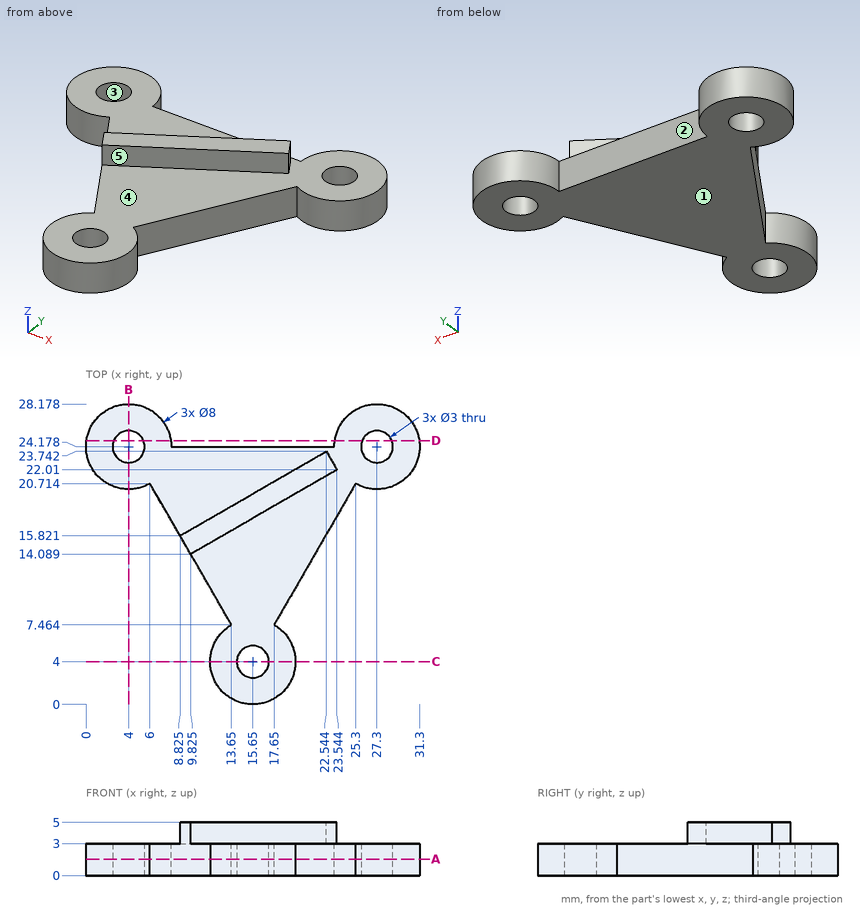
Geometry: see drawing. Coordinates: mm, zero at the bounding-box minimum. A direction names the side the tool comes from. Coordinates: 2 decimals unless noted, no trailing zeros. Loops run counter-clockwise (first coordinate to the right, second up) from the corner with the lowest first, then second, coordinate; pieces in that order, holes last. Notation, with made-up numbers: (50, 11) -> (83, 11) arc R3 ccw to (83, 16) -> close; hole circle Ø10 at (-30.75, 28). An arc over 180 degrees is marked (long way). Use a Markdown table: item, result.
1) Pull-direction query (X, two-part tool) for the marked faces 3, 4 and 5; classes: released by +X, released by -X, zero draft, split by the parting line, or undercut.
Results found:
| item | result |
|---|---|
| face 3 | undercut |
| face 4 | zero draft |
| face 5 | released by +X |
2) Cut plane C-C (y = 4). Return the cut outline in (x, z).
Results found:
| item | result |
|---|---|
| outline | (11.65, 0) -> (14.15, 0) -> (14.15, 3) -> (11.65, 3) -> close; (17.15, 0) -> (19.65, 0) -> (19.65, 3) -> (17.15, 3) -> close |
3) Cut plane A-A (z = 1.55). Give the number of separate pieces and of enclosed holes in the cut face.
Results found:
| item | result |
|---|---|
| separate pieces | 1 |
| enclosed holes | 3 |
4) Cut plane D-D (y = 24.75). Return the cut outline in (x, z).
Results found:
| item | result |
|---|---|
| outline | (0.04, 0) -> (2.61, 0) -> (2.61, 3) -> (0.04, 3) -> close; (5.39, 0) -> (7.96, 0) -> (7.96, 3) -> (5.39, 3) -> close; (23.34, 0) -> (25.91, 0) -> (25.91, 3) -> (23.34, 3) -> close; (28.69, 0) -> (31.26, 0) -> (31.26, 3) -> (28.69, 3) -> close |
5) Contact query for flat-ended pins moving along their axis: pin 1 (1.5 mm diameter, centred on y = 22, z = 1.5, fed in from +X); pin 2 (3 mm diameter, centred on y = 8.5, z = 3.5, fed in from +X) (1 decimal). Output: stop coordinate, or through.
Results found:
| item | result |
|---|---|
| pin 1 | stops at x = 31.04 |
| pin 2 | stops at x = 19.1 |
6) Material intervals for line 1 along Y through (x, z) = (27.3, 1.85); line 2 along X through (y, z) = (25.5, 2) (1 decimal); line 3 along Z through (x, y) = (16, 20.25), sorted ascending. Write a range as from..to.
Results found:
| item | result |
|---|---|
| line 1 | y = 20.18..22.68, 25.68..28.18 |
| line 2 | x = 0.2..3.3, 4.7..7.8, 23.5..26.6, 28..31.1 |
| line 3 | z = 0..3 |
7) Access query for the marked faces 1 and 2. Directions: +Z, -Z, +X, -X, +Y, -Y. A direction counts if a zero-diameter tool reaches every point of the face in a straight line with its end or side. Return the directions, or none.
Results found:
| item | result |
|---|---|
| face 1 | -Z, +X, -X, +Y, -Y |
| face 2 | +Z, -Z, +Y |
8) Cut plane B-B (x = 4). Return the cut outline in (y, z), then the cut area to 3 significant figures.
Results found:
| item | result |
|---|---|
| outline | (20.18, 0) -> (22.68, 0) -> (22.68, 3) -> (20.18, 3) -> close; (25.68, 0) -> (28.18, 0) -> (28.18, 3) -> (25.68, 3) -> close |
| area | 15.0 mm2 |
